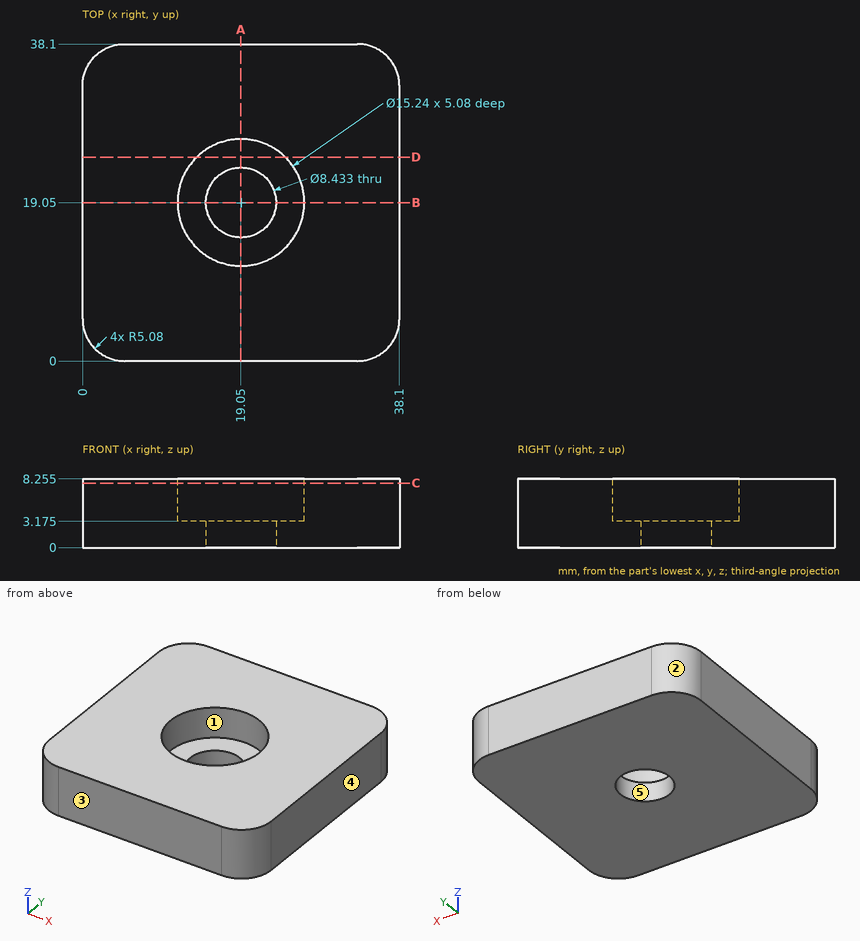
Part print with two shaded views. Sizes in mm from the minimum x, y, z corner. A direction names the side the tool comes from. Round coordinates to 2 decimals unless told otherwise and drop trailing zeros. Loops run counter-clockwise (first coordinate to the right, second up) from the corner with the lowest first, then second, coordinate; pieces in that order, holes last.
1. Slice it at A-A (x = 19.05). Give the cut face in (y, z) (1 decimal).
Solutions:
outline: (0, 0) - (14.8, 0) - (14.8, 3.2) - (11.4, 3.2) - (11.4, 8.3) - (0, 8.3) - close; (23.3, 0) - (38.1, 0) - (38.1, 8.3) - (26.7, 8.3) - (26.7, 3.2) - (23.3, 3.2) - close
2. Two-plate mould, pull along Y, no slides. Class the marked faces 3, 4 and 5: pulls with the +Y half, pulls with the -Y half, needs draft (parallel to the pull), parting line crosses it, or undercut.
Solutions:
face 3: pulls with the -Y half
face 4: needs draft
face 5: undercut
3. Slice it at C-C (z = 7.75). Give the cut face in (x, y), and give its area (3 significant figures).
Solutions:
outline: (0, 5.08) arc R5.08 ccw to (5.08, 0) - (33.02, 0) arc R5.08 ccw to (38.1, 5.08) - (38.1, 33.02) arc R5.08 ccw to (33.02, 38.1) - (5.08, 38.1) arc R5.08 ccw to (0, 33.02) - close; hole circle Ø15.24 at (19.05, 19.05)
area: 1,250 mm2
4. Drill centre lines: line 1 along Y through (x, z) = (19.05, 6.25); line 2 along Y through (x, z) = (19.05, 1.9); line 3 along Z through (x, y) = (18.5, 12) (3 decimals). Where is each one in solid material? Low to high.
Solutions:
line 1: y = 0 to 11.43, 26.67 to 38.1
line 2: y = 0 to 14.83, 23.27 to 38.1
line 3: z = 0 to 3.175
5. Slice it at D-D (y = 24.5). Give the cut face in (x, z) (1 decimal).
Solutions:
outline: (0, 0) - (38.1, 0) - (38.1, 8.3) - (24.4, 8.3) - (24.4, 3.2) - (13.7, 3.2) - (13.7, 8.3) - (0, 8.3) - close
6. Flat gauge pin, fed straight in: pin 1 (7.5 mm diameter, centred on x = 19.5, y = 16, fed in from +Z) (3 decimals). Where does the tip first touch, or does it go through?
Solutions:
pin 1: stops at z = 3.175
7. 3-axis set-ups, long thin cutter, end or side, ignore diameter. For the marked faces 1 and 2: which of +Z, -Z, +X, -X, +Y, -Y reach the whole face in a straight line?
Solutions:
face 1: +Z
face 2: +Z, -Z, -X, +Y
